Input: part model. Units: mm. Frame: model coordinates. Face numbers are marked on the shaded views. A direction names the side the tool comes from. Give positions to 0.01 mm unless a question says otherwise; leave off trailing zeros. Loops run counter-clockwise (first coordinate to the right, second up) from the corner with the lowest first, then second, coordinate; pieces in that order, holes last. Notation, with made-up numbers: (-18.75, 44.25) - (39.25, 44.25) arc R8 cw to (39.25, 49.25) - close; hole circle Ø10 at (2, 77.25). An arc over 180 degrees is marked (long way). Answer as a JSON object with one key per item and string values. Group by question number.
(1) Access query for the marked faces 1 and 2. Directions: +Z, -Z, +X, -X, +Y, -Y. A direction counts if a zero-diameter tool reaches every point of the face in a straight line with its end or side. Return the directions, or none.
(2) Material intervals for L1, parallel to Z at x = 1.75, y = -0.85; L2, parallel to X at y = 0.1, z = -1.25; L3, parallel to Y at x = -1.3, z = -12.75, sorted ascending.
(3) Pin query (flat end, axial travel): P1, Ø3, axis at x = 2, z = -16, coming from the +Y side; P2, Ø2, axis at x = 2, z = -16, coming from the +Y side; P3, Ø1, axis at y = 1.5, z = -16, coming from the +X side. Return the tip coordinate at first contact, or that it passes through.
(4) Section query A-A (z = -16.5). Return loops of the section in (x, y), plus the area to 3 significant figures.
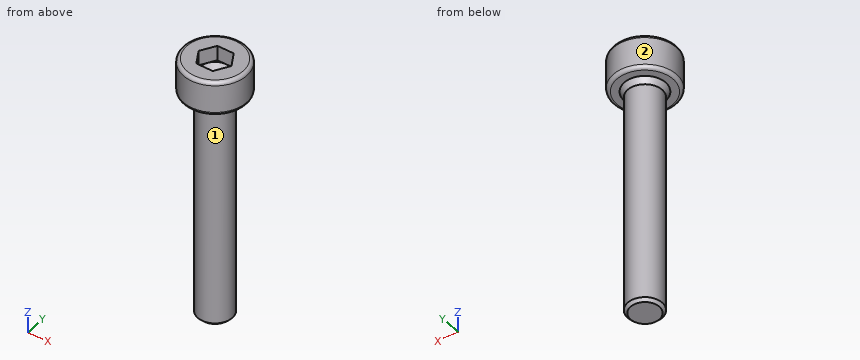
Solid Edge part; units mm, degrees
sketch "Sketch1" plane through (0, 0, 0) normal (0, -1, 0) x (1, 0, 0)
  line L0 (2.75, 3) -> (2.75, 0)
  line L1 (2.75, 0) -> (1.8, 0)
  line L2 (1.8, 0) -> (1.5, -0.5196)
  line L3 (1.5, -0.5196) -> (1.5, -20)
  line L4 (1.5, -20) -> (0, -20)
  line L5 (1.25, 1.7) -> (0, 0.9783)
  line L6 (1.25, 3) -> (1.25, 1.7)
  line L7 (2.75, 3) -> (1.25, 3)
revolve "RevolvedProtrusion1" add sketch "Sketch1" angle 360 about axis through (0, 0, -6) along (0, 0, 1)
cosmetic_thread "Thread1"
chamfer "Chamfer_1" distance 0.25 angle 45 1 edges at (-1.5, 0, -20)
fillet "Round_1" radius 0.3 2 edges at (-2.75, 0, 0) (-2.75, 0, 3)
sketch "Sketch2" plane through (0, 0, 3) normal (0, 0, 1) x (0, 1, 0)
  line L0 (-1.25, 0.7217) -> (-1.25, -0.7217)
  line L1 (0, -1.4434) -> (-1.25, -0.7217)
  line L2 (1.25, -0.7217) -> (0, -1.4434)
  line L3 (1.25, 0.7217) -> (1.25, -0.7217)
  line L4 (0, 1.4434) -> (1.25, 0.7217)
  line L5 (-1.25, 0.7217) -> (0, 1.4434)
extrude "Cutout1" cut sketch "Sketch2" against normal up to vertex (1.3 mm away)
properties material "Galvanized steel"
Recorded:
{
 "1": {"face 1": "-Z", "face 2": "+Z, -Z"},
 "2": {"L1": "z = 0 to 3", "L2": "x = -1.5 to 1.5", "L3": "y = -0.75 to 0.75"},
 "3": {"P1": "stops at y = 1.41", "P2": "stops at y = 1.12", "P3": "stops at x = 1.12"},
 "4": {"outline": "circle Ø3 at (0, 0)", "area": "7.07 mm^2"}
}
